Can you work these out from the model? Positions are in its coordinate system, mm. Face numbers are marked on the shaded views. Round coordinates to 2 decimals unless told otherwise and drop trailing zeros. Order: outer loops, then holes, each group sorted by start corner. A loop starts at its lowest first (then second) coordinate and runs counter-clockwise, first axis right, second up. Notation, with made-up numbers: (17, 3.5) -> (63, 3.5) arc R8 ccw to (63, 8.5) -> close; hole circle Ø6 at (47.25, -39.5). An arc over 180 degrees is marked (long way). Use a Markdown table: item, result. Add a question column.
Q1. If we section it at C-C on y = -17.5: List the corners of the cut face in (x, z) for me, plus the area to 3 significant figures.
Q2. If we section it at D-D on z = 1.3: List the corners of the cut face in (x, y) for me (3 decimals).
Q3. If we section it at B-B on y = 10.45: List the corners of the cut face in (x, z) for me, plus the area to 3 significant figures.
Q4. If we section it at A-A on x = 0: List the corners of the cut face in (y, z) for me, plus the area to 3 significant figures.
Q5. I'm going to push a flat-ended pin straight in: pin 1 Ø0.5 at (y, z) = (-15, 3) entering from -X. Where does the tip first touch, or does it pass through?
Q6. I need wall thicknesses on line 1 along X through (y, z) = (0, 0.9); line 2 along Y through (x, z) = (9.5, 1.65); line 3 along X through (y, z) = (-1, 2.1). Which ranges of each line are inside material? Lowest first, please. Write a range as [from, to].
Q7. We'd pull the mould along X, two halves only. Please class the marked faces 1, 2 and 3: +X half, -X half, draft (parallel to the pull), parting line (faces both ways), or undercut.
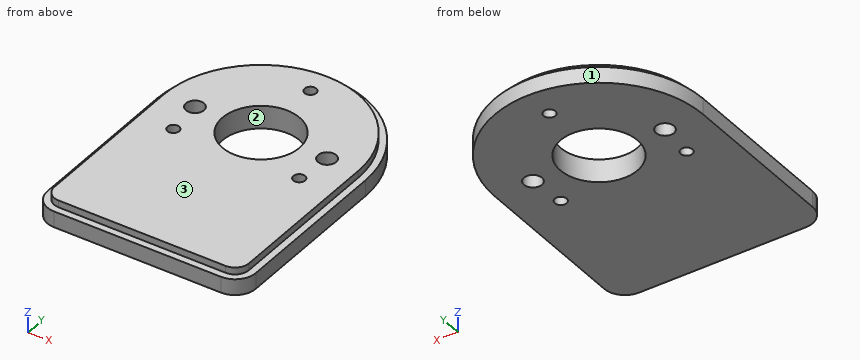
Autodesk Inventor part; units mm, degrees
ref_plane "YZ Plane" through (0, 0, 0) normal (1, 0, 0) x (0, 1, 0)
ref_plane "XZ Plane" through (0, 0, 0) normal (0, 1, 0) x (-1, 0, 0)
ref_plane "XY Plane" through (0, 0, 0) normal (0, 0, 1) x (1, 0, 0)
sketch "スケッチ1" plane through (0, 0, 0) normal (0, 0, 1) x (1, 0, 0)
  line L0 (-15, 0.0806) -> (15, 0.0806)
  line L1 (15, 0.0806) -> (15, -26.1194)
  line L2 (15, -26.1194) -> (-15, -26.1194)
  line L3 (-15, -26.1194) -> (-15, 0.0806)
  circle A0 centre (0, 0) radius 15.0002
  dimension "d0" = 30
  dimension "d1" = 15
  dimension "d2" = 26.2
extrude "押し出し1" add sketch "スケッチ1" along normal blind 3.3
sketch "スケッチ2" plane through (0, 0, 3.3) normal (0, 0, 1) x (1, 0, 0)
  arc A0 (15, -0.0806) -> (-15, -0.0806) centre (0, 0) ccw
  circle A1 centre (0, 0) radius 9.5
  point P0 (-9.5, 0)
  point P1 (9.5, 0)
  dimension "d5" = 19
hole "Hole1" at (-9.5, 0, 3.3) at (9.5, 0, 3.3) direction (0, 0, -1) diameter 2.6 depth 10
sketch "スケッチ3" plane through (0, 0, 3.3) normal (0, 0, 1) x (1, 0, 0)
  arc A0 (15, -0.0806) -> (-15, -0.0806) centre (0, 0) ccw
hole "Hole2" at (0, 0, 3.3) direction (0, 0, -1) diameter 11.1 depth 10 tip angle 118
sketch "スケッチ4" plane through (0, 0, 3.3) normal (0, 0, 1) x (1, 0, 0)
  arc A0 (15, -0.0806) -> (-15, -0.0806) centre (0, 0) ccw
  line L0 (-15, -26.1194) -> (-15, -0.0806)
  line L1 (15, -26.1194) -> (-15, -26.1194)
  line L2 (15, -0.0806) -> (15, -26.1194)
  line L3 (-14, -0.0806) -> (14, -0.0806)
  line L4 (14, -0.0806) -> (14, -25.1194)
  line L5 (14, -25.1194) -> (-14, -25.1194)
  line L6 (-14, -25.1194) -> (-14, -0.0806)
  circle A1 centre (0, 0) radius 14.0002
  dimension "d20" = 1
  dimension "d21" = 1
  dimension "d22" = 1
extrude "押し出し2" cut sketch "スケッチ4" against normal blind 1
fillet "フィレット1" radius 3 2 edges at (15, -26.1194, 1.15) (-15, -26.1194, 1.15)
fillet "フィレット2" radius 2 2 edges at (14, -25.1194, 2.8) (-14, -25.1194, 2.8)
sketch "スケッチ5" plane through (0, 0, 3.3) normal (0, 0, 1) x (1, 0, 0)
  circle A0 centre (0, 0) radius 5.55
  circle A1 centre (0, 0) radius 10.45
  point P0 (0, 10.45)
  point P1 (-9.05, -5.225)
  point P2 (9.05, -5.225)
  dimension "d27" = 20.9
  dimension "d30" = 360
hole "Hole3" at (0, 10.45, 3.3) at (-9.05, -5.225, 3.3) at (9.05, -5.225, 3.3) direction (0, 0, -1) diameter 1.7 end through all
equation "\"d22\" = d21"
properties part number "HEDS-5500_A"
Answer below:
| question | item | result |
|---|---|---|
| 1 | outline | (-15, 0) -> (15, 0) -> (15, 2.3) -> (14, 2.3) -> (14, 3.3) -> (-14, 3.3) -> (-14, 2.3) -> (-15, 2.3) -> close |
| 1 | area | 97.0 mm² |
| 2 | outline | (-15, -23.119) arc R3 ccw to (-12, -26.119) -> (12, -26.119) arc R3 ccw to (15, -23.119) -> (15, 0.081) arc R15 ccw to (-15, 0.081) -> close; hole circle Ø2.6 at (-9.5, 0); hole circle Ø1.7 at (-9.05, -5.225); hole circle Ø11.1 at (0, 0); hole circle Ø1.7 at (0, 10.45); hole circle Ø1.7 at (9.05, -5.225); hole circle Ø2.6 at (9.5, 0) |
| 3 | outline | (-10.76, 0) -> (-0.85, 0) -> (-0.85, 3.3) -> (-9.32, 3.3) -> (-9.32, 2.3) -> (-10.76, 2.3) -> close; (0.85, 0) -> (10.76, 0) -> (10.76, 2.3) -> (9.32, 2.3) -> (9.32, 3.3) -> (0.85, 3.3) -> close |
| 3 | area | 62.5 mm² |
| 4 | outline | (-26.12, 0) -> (-5.55, 0) -> (-5.55, 3.3) -> (-25.12, 3.3) -> (-25.12, 2.3) -> (-26.12, 2.3) -> close; (5.55, 0) -> (9.6, 0) -> (9.6, 3.3) -> (5.55, 3.3) -> close; (11.3, 0) -> (15, 0) -> (15, 2.3) -> (14, 2.3) -> (14, 3.3) -> (11.3, 3.3) -> close |
| 4 | area | 91.5 mm² |
| 5 | pin 1 | x = -14 |
| 6 | line 1 | [-15, -10.8], [-8.2, -5.55], [5.55, 8.2], [10.8, 15] |
| 6 | line 2 | [-26.12, -5.95], [-4.5, -1.3], [1.3, 11.61] |
| 6 | line 3 | [-15, -10.33], [-8.67, -5.46], [5.46, 8.67], [10.33, 15] |
| 7 | face 1 | parting line |
| 7 | face 2 | undercut |
| 7 | face 3 | draft |
